Design review of the part built by this model. Coordinates are the model's own, in mm. Coordinates: 2 decimals unless noted, no trailing zeros. Order: outer loops, then holes, each group sorted by start corner. A loop starts at its lowest first (then second) coordinate and runs counter-clockwise, first axis right, second up. Notation, with made-up numbers: M -20.5,13.5 L -12.5,13.5 A18 ccw -12.5,25.5 Z; hole C 68.5,14.25 d8. An arc over 180 degrees is marked long. Answer in a Markdown table with one row per item.
from build123d import *

# Parameters (mm, degrees)
SKETCH3_R                      = 1.6
SKETCH3_R_2                    = 3
BOSS_EXTRUDE1_DEPTH            = 3
F_3_0MM_DOWEL_HOLE1_AT_2_COUNT = 2
F_3_0MM_DOWEL_HOLE1_AT_2_PITCH = 28
F_5_0MM_DOWEL_HOLE1_D          = 5
F_5_0MM_DOWEL_HOLE1_DEPTH      = 5
F_5_0MM_DOWEL_HOLE1_TIP        = 1.502151548
SKETCH12_R                     = 1.5
CUT_EXTRUDE1_DEPTH             = 151.029997001
SKETCH13_W                     = 8
SKETCH13_H                     = 30
CUT_EXTRUDE2_DEPTH             = 3


with BuildPart() as part:
    # Sketch3 → Boss-Extrude1 (new body)
    with BuildSketch(Plane(origin=(0, 0, 0), x_dir=(1, 0, 0), z_dir=(0, 1, 0))):
        Polygon((-70, 90), (80, 90), (120, 50), (120, -50), (80, -90), (-70, -90), (-110, -50), (-110, 50), align=None)
        with Locations(Location((-99, 55, 0), (0, 0, 90))):
            Circle(SKETCH3_R, mode=Mode.SUBTRACT)
        with Locations(Location((-99, -55, 0), (0, 0, 270))):
            Circle(SKETCH3_R, mode=Mode.SUBTRACT)
        with Locations(Location((43.5, -55, 0), (0, 0, 270))):
            Circle(SKETCH3_R_2, mode=Mode.SUBTRACT)
        with Locations(Location((43.5, -75, 0), (0, 0, 270))):
            Circle(SKETCH3_R_2, mode=Mode.SUBTRACT)
        with Locations(Location((43.5, 75, 0), (0, 0, 90))):
            Circle(SKETCH3_R_2, mode=Mode.SUBTRACT)
        with Locations(Location((43.5, 55, 0), (0, 0, 90))):
            Circle(SKETCH3_R_2, mode=Mode.SUBTRACT)
        with Locations(Location((-35, 10, 0), (0, 0, 270))):
            Circle(SKETCH3_R_2, mode=Mode.SUBTRACT)
        with Locations(Location((-35, -10, 0), (0, 0, 90))):
            Circle(SKETCH3_R_2, mode=Mode.SUBTRACT)
        with Locations(Location((50, -22, 0), (0, 0, 270))):
            Circle(SKETCH3_R, mode=Mode.SUBTRACT)
        with Locations(Location((95, -8.5, 0), (0, 0, 270))):
            Circle(SKETCH3_R, mode=Mode.SUBTRACT)
        with Locations(Location((22, 22, 0), (0, 0, 270))):
            Circle(SKETCH3_R, mode=Mode.SUBTRACT)
        with Locations(Location((50, 22, 0), (0, 0, 270))):
            Circle(SKETCH3_R, mode=Mode.SUBTRACT)
        with Locations(Location((95, 8.5, 0), (0, 0, 90))):
            Circle(SKETCH3_R, mode=Mode.SUBTRACT)
        with Locations(Location((22, -22, 0), (0, 0, 270))):
            Circle(SKETCH3_R, mode=Mode.SUBTRACT)
        with Locations(Location((-75, -70, 0), (0, 0, 270))):
            Circle(SKETCH3_R, mode=Mode.SUBTRACT)
        with Locations(Location((2, -70, 0), (0, 0, 270))):
            Circle(SKETCH3_R, mode=Mode.SUBTRACT)
        with Locations(Location((2, 70, 0), (0, 0, 90))):
            Circle(SKETCH3_R, mode=Mode.SUBTRACT)
        with Locations(Location((-75, 70, 0), (0, 0, 90))):
            Circle(SKETCH3_R, mode=Mode.SUBTRACT)
    extrude(amount=BOSS_EXTRUDE1_DEPTH)

    # Sketch9 → Ø3.0mm Dowel Hole1 (revolve, cut)
    with BuildSketch(Plane(origin=(-21, 0, -86.5), x_dir=(0, 0, -1), z_dir=(1, 0, 0))):
        Polygon((0, 0), (0, 5.901290929), (1.5, 5), (1.5, 0), align=None)
    f_3_0mm_dowel_hole1 = revolve(axis=Axis((-21, -6.35, -86.5), (0, 1, 0)), mode=Mode.SUBTRACT)

    # Ø3.0mm Dowel Hole1 at 2: Ø3.0mm Dowel Hole1 ×2
    with Locations(*[(-i * F_3_0MM_DOWEL_HOLE1_AT_2_PITCH, 0, 0) for i in range(1, F_3_0MM_DOWEL_HOLE1_AT_2_COUNT)]):
        add(f_3_0mm_dowel_hole1, mode=Mode.SUBTRACT)

    # Mirror3: Ø3.0mm Dowel Hole1 across plane
    add(f_3_0mm_dowel_hole1.mirror(Plane.XY), mode=Mode.SUBTRACT)

    # Mirror3 copy 1 sketch → Mirror3 copy 1 (revolve, cut)
    with BuildSketch(Plane(origin=(-49, 0, 86.5), x_dir=(0, 0, 1), z_dir=(1, 0, 0))):
        Polygon((0, 0), (0, -5.901290929), (1.5, -5), (1.5, 0), align=None)
    revolve(axis=Axis((-49, -6.35, 86.5), (0, -1, 0)), mode=Mode.SUBTRACT)

    # Ø5.0mm Dowel Hole1
    with Locations(Plane(origin=(110, 0, -20), x_dir=(0, 0, -1), z_dir=(0, -1, 0))):
        with Locations((0, 0), (-40, 0)):
            Hole(F_5_0MM_DOWEL_HOLE1_D / 2, depth=F_5_0MM_DOWEL_HOLE1_DEPTH)
            with Locations((0, 0, -(F_5_0MM_DOWEL_HOLE1_DEPTH + F_5_0MM_DOWEL_HOLE1_TIP / 2))):  # 118° drill point
                Cone(0, F_5_0MM_DOWEL_HOLE1_D / 2, F_5_0MM_DOWEL_HOLE1_TIP, mode=Mode.SUBTRACT)

    # Sketch12 → Cut-Extrude1 (cut, through all)
    with BuildSketch(Plane(origin=(0, 3, 0), x_dir=(1, 0, 0), z_dir=(0, 1, 0))):
        with Locations(Location((-61, -86.5, 0), (0, 0, 270))):
            Circle(SKETCH12_R)
        with Locations(Location((-9, -86.5, 0), (0, 0, 270))):
            Circle(SKETCH12_R)
        with Locations(Location((-61, 86.5, 0), (0, 0, 90))):
            Circle(SKETCH12_R)
        with Locations(Location((-9, 86.5, 0), (0, 0, 90))):
            Circle(SKETCH12_R)
    extrude(amount=-CUT_EXTRUDE1_DEPTH, mode=Mode.SUBTRACT)

    # Sketch13 → Cut-Extrude2 (cut)
    with BuildSketch(Plane(origin=(0, 0, 0), x_dir=(-1, 0, 0), z_dir=(0, -1, 0))):
        with Locations((82.5, 0)):
            Rectangle(SKETCH13_W, SKETCH13_H)
    extrude(amount=-CUT_EXTRUDE2_DEPTH, mode=Mode.SUBTRACT)


solid = part.part
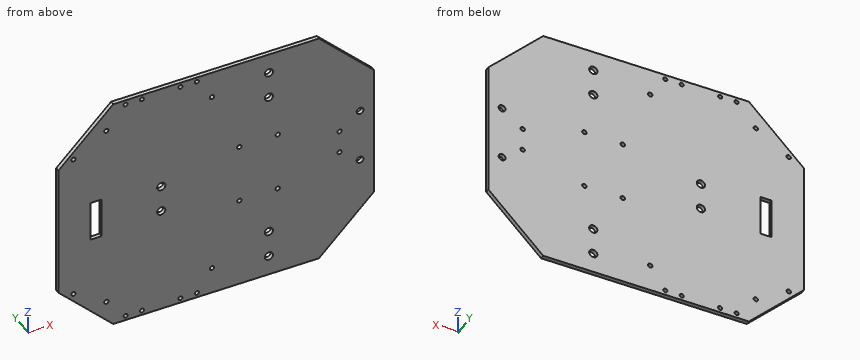
(1) Add section A-A, the plane x = 110. Give the boundary of the cut face in (y, z).
Return value:
| item | result |
|---|---|
| outline | M 0,-60 L 3,-60 L 3,-22.5 L 0,-22.5 Z; M 0,-17.5 L 3,-17.5 L 3,17.5 L 0,17.5 Z; M 0,22.5 L 3,22.5 L 3,60 L 0,60 Z |
(2) For line 1 along Z through (x, y) = (-49, 1.55); line 2 along Z through (x, y) = (-75, 0.9); line 3 along X through (y, z) = (1.7, 86.5), list the stretches that pass through material, from the lowest coordinate up. Write a range as from..to.
Return value:
| item | result |
|---|---|
| line 1 | z = -90..-88, -85..85, 88..90 |
| line 2 | z = -85..-71.6, -68.4..68.4, 71.6..85 |
| line 3 | x = -73.5..-62.5, -59.5..-50.5, -47.5..-22.5, -19.5..-10.5, -7.5..83.5 |
(3) Add section B-B, the plane y = 2.2. Give the number of separate pieces and of enclosed holes in the cut face, and give its area (3 significant figures).
Return value:
| item | result |
|---|---|
| separate pieces | 1 |
| enclosed holes | 29 |
| area | 37,600 mm2 |
